from build123d import *

# Parameters (mm, degrees)
F1_DEPTH    = 30
F2_T1_DEPTH = 90
F2_T4_ANGLE = 236.2626685885
F2_T6_ANGLE = 236.2626685885


# Not quite as in the source:
# - a fillet or chamfer that OpenCascade refuses, or shapes differently, is made with other operations: its cross-section is extruded or revolved along the edge and cut away or added


with BuildPart() as f1:
    # F0 (on Front) → F1 (new body)
    with BuildSketch(Plane.XZ):
        with BuildLine():
            Line((0, 35), (0, 0))
            Line((0, 0), (7, 0))
            ThreePointArc((7, 0), (32.5, 25.5), (58, 0))
            Line((58, 0), (65, 0))
            Line((65, 0), (65, 35))
            Line((65, 35), (0, 35))
        make_face()
    extrude(amount=F1_DEPTH)

    # F2: fillet of radius 5 on 4 edges, made by hand

    # F2_s2 → F2_t1 (cut)
    with BuildSketch(Plane.YZ.offset(-12.5)):
        with BuildLine():
            ThreePointArc((-25, 35), (-28.5355339059, 33.5355339059), (-30, 30))
            Line((-30, 30), (-30, 35))
            Line((-30, 35), (-25, 35))
        make_face()
        with BuildLine():
            ThreePointArc((-5, 35), (-1.4644660941, 33.5355339059), (0, 30))
            Line((0, 30), (0, 35))
            Line((0, 35), (-5, 35))
        make_face()
    extrude(amount=F2_T1_DEPTH, mode=Mode.SUBTRACT)

    # F2_s3 → F2_t4 (revolve, cut)
    with BuildSketch(Plane(origin=(7.2249714164, 0, -13.5133770415), x_dir=(0, 1, 0), z_dir=(0.4714942341, 0, -0.881869144))):
        with BuildLine():
            ThreePointArc((-25, 3.1607471809), (-28.5355339059, 1.6962810868), (-30, -1.8392528191))
            Line((-30, -1.8392528191), (-30, 3.1607471809))
            Line((-30, 3.1607471809), (-25, 3.1607471809))
        make_face()
    revolve(axis=Axis((32.5, -30, 0), (0, 1, 0)), revolution_arc=F2_T4_ANGLE, mode=Mode.SUBTRACT)

    # F2_s5 → F2_t6 (revolve, cut)
    with BuildSketch(Plane(origin=(7.2249714164, 0, -13.5133770415), x_dir=(0, 1, 0), z_dir=(0.4714942341, 0, -0.881869144))):
        with BuildLine():
            ThreePointArc((-5, 3.1607471809), (-1.4644660941, 1.6962810868), (0, -1.8392528191))
            Line((0, -1.8392528191), (0, 3.1607471809))
            Line((0, 3.1607471809), (-5, 3.1607471809))
        make_face()
    revolve(axis=Axis((32.5, 0, 0), (0, 1, 0)), revolution_arc=F2_T6_ANGLE, mode=Mode.SUBTRACT)


solid = f1.part
Design review of the part built by this model. Coordinates are the model's own, in mm. Coordinates: 2 decimals unless noted, no trailing zeros. Write each loop counter-clockwise with the first axis right and the second up, starting at its lowest first coordinate (ties: lowest second). Pieces come first, ordered by that corner, then holes. Notation, with made-up numbers: (41, 19) -> (66, 19) arc R13 ccw to (66, 42) -> close; hole circle Ø6 at (74, 61). An arc over 180 degrees is marked (long way). Write each question's results on one line, items separated by ' | '. Start each with the question number.
(1) Clearance check with flat-ended pins moving along their axes: P1, Ø3, axis at y = -21, z = 17.5, coming from the -X side; P2, Ø1.5, axis at x = 22, y = -23.5, coming from the -Z side; P3, Ø4, axis at x = 34.5, y = -13, coming from the -Z side; P4, Ø3, axis at x = 58.5, z = 4, coming from the -Y side. State where each tip first meets the part, or that it passes through.
(2) The part is to be moulded in two halves that separate along X. For faces 1 (the face through (65, -15, 17)), 2 (the face through (61, -15, 0)), 3 (the face through (31.939, -14.86, 25.494)), 4 (the face through (0, -15, 18)), say which applies: pulls with the +X half, pulls with the -X half, needs draft (parallel to the pull), parting line crosses it, or undercut.
(3) For line 1 along X through (y, z) = (-18, 6.5); line 2 along X through (y, z) = (-2, 6.5); line 3 along Z through (x, y) = (51, -13.5), list the stretches that pass through material, from the lowest coordinate up. Write a range as from..to.
(4) Take a section at B-B on y = -28. Write out the cut boundary in (x, z).
(5) Take a section at A-A on y = -24. Write out the cut boundary in (x, z), and give its area (3 significant figures).
Results found:
1) P1: stops at x = 0 | P2: stops at z = 22.88 | P3: stops at z = 25.18 | P4: stops at y = -29.21
2) face 1: pulls with the +X half | face 2: needs draft | face 3: undercut | face 4: pulls with the -X half
3) line 1: x = 0..7.84, 57.16..65 | line 2: x = 0..6.81, 58.19..65 | line 3: z = 17.55..35
4) outline: (0, 0) -> (6, 0) arc R26.5 cw to (59, 0) -> (65, 0) -> (65, 34) -> (0, 34) -> close
5) outline: (0, 0) -> (7, 0) arc R25.5 cw to (58, 0) -> (65, 0) -> (65, 35) -> (0, 35) -> close | area: 1,250 mm2
